Can you work these out from the model? Positions are in its coordinate system, mm. A direction names the side the tool comes from. Give positions to 0.01 mm unless a question says otherwise; leave off trailing zeros. Write each loop counter-clockwise with the first axis right and the second up, starting at its lowest first coordinate (ties: lowest second). Pieces come first, ordered by that corner, then holes. Notation, with made-up numbers: (-9, -24) -> (14, -24) arc R13 ccw to (14, -7) -> close; hole circle Ø4 at (7, 39). An arc over 180 degrees is marked (long way). One line per item, written item: value.
from build123d import *

# Parameters (mm, degrees)
SKETCH_1_R          = 10.5
EXTRUDE_1_DEPTH     = 35
FILLET_1_R          = 7
SKETCH_2_W          = 7.958584752
SKETCH_2_H          = 21.543065623
CUT_EXTRUDE_2_DEPTH = 20
SKETCH_3_R          = 2.5
CUT_EXTRUDE_3_DEPTH = 41.093640507


with BuildPart() as part:
    # Эскиз1 → Вытянуть1 (new body)
    with BuildSketch(Plane(origin=(0, 0, 0), x_dir=(1, 0, 0), z_dir=(0, 1, 0))):
        with Locations(Location((0, 0, 0), (0, 0, 270))):
            Circle(SKETCH_1_R)
    extrude(amount=EXTRUDE_1_DEPTH)

    # Скругление1
    fillet_1_edges = [part.edges().sort_by_distance(p)[0] for p in [
        (0, 35, -10.5),
    ]]
    fillet(fillet_1_edges, radius=FILLET_1_R)

    # Эскиз2 → Вытянуть2 (cut, symmetric)
    with BuildSketch(Plane.XY):
        with Locations((9.979292376, 27.395051325)):
            Rectangle(SKETCH_2_W, SKETCH_2_H)
        with Locations((-9.979292376, 27.395051325)):
            Rectangle(SKETCH_2_W, SKETCH_2_H)
    extrude(amount=CUT_EXTRUDE_2_DEPTH, both=True, mode=Mode.SUBTRACT)

    # Эскиз3 → Вытянуть3 (cut, through all)
    with BuildSketch(Plane(origin=(6, 0, 0), x_dir=(0, 0, -1), z_dir=(1, 0, 0))):
        with Locations(Location((0, 28.011489149, 0), (0, 0, 90))):
            Circle(SKETCH_3_R)
    extrude(amount=-CUT_EXTRUDE_3_DEPTH, mode=Mode.SUBTRACT)


solid = part.part
1) Will these pins go through, and if not, where does the flat tip stop? pin 1 (1.5 mm diameter, centred on x = 4.5, y = 31.5, fed in from +Z); pin 2 (1.4 mm diameter, centred on x = -7.5, z = -1.5, fed in from +Y); pin 3 (6.5 mm diameter, centred on y = 28.01, z = 0, fed in from +X).
Answer list:
pin 1: stops at z = 9
pin 2: stops at y = 16.62
pin 3: stops at x = 6
2) If we section it at B-B (x = 6.75): Write out the boundary of the cut face in (y, z), and give its area (3 significant figures).
Answer list:
outline: (0, -8.04) -> (16.62, -8.04) -> (16.62, 8.04) -> (0, 8.04) -> close
area: 267 mm^2
3) If we section it at A-A (y = 6.5): Write out the boundary of the cut face in (x, z), and give its area (3 significant figures).
Answer list:
outline: circle Ø21 at (0, 0)
area: 346 mm^2
4) For faces 1 (the face through (0, 0, 0)), 2 (the face through (-6, 25, 0)), 3 (the face through (6, 25, 0)), which set-ups out of +Z, -Z, +X, -X, +Y, -Y let a thin tool reach every point of the face, with its end or its side?
Answer list:
face 1: +Z, -Z, +X, -X, -Y
face 2: +Z, -Z, -X, +Y
face 3: +Z, -Z, +X, +Y
5) We'd pull the mould along Z, two halves only. Please class faces 4 (the face through (3.2, 10.7, 10)), 5 (the face through (0.08, 30.32, -0.96)), 6 (the face through (0, 35, 0)): released by +Z, released by -Z, zero draft, split by the parting line, or undercut.
Answer list:
face 4: split by the parting line
face 5: undercut
face 6: zero draft
6) If we section it at C-C (y = 24): Write out the boundary of the cut face in (x, z).
Answer list:
outline: (-6, -8.62) arc R10.5 ccw to (6, -8.62) -> (6, 8.62) arc R10.5 ccw to (-6, 8.62) -> close
7) I need wall thicknesses on L1, parallel to X at y = 26, z = 4; L2, parallel to Z at x = -4.75, y = 28; L3, parallel to Y at x = -7, z = 1.5. Which ranges of each line are inside material? Lowest first, please.
Answer list:
L1: x = -6 to 6
L2: z = -9.36 to -2.5, 2.5 to 9.36
L3: y = 0 to 16.62
